Work out the finished part from the listing and answer in its coordinate system (mm). Face numbers are marked on the shaded views. A direction names the side the tool comes from. Give positions to 0.01 mm unless a question says otherwise; leave off trailing zeros. Order: outer loops, then holes, each group sorted by start corner. A loop starts at its lowest first (then second) coordinate and runs counter-clockwise, first axis right, second up. Notation, with made-up numbers: (79, 22) - (107, 22) arc R21 cw to (107, 53) - close; hole circle Ø7 at (60, -16). An arc over 180 degrees is marked (long way). Put each result on its own line as item: value.
```python
from build123d import *

# Parameters (mm, degrees)
F1_DEPTH = 25.4


with BuildPart() as f1:
    # F0 (on Right) → F1 (new body)
    with BuildSketch(Plane.YZ):
        with BuildLine():
            Line((-2.9690999484, -55.5171445012), (-30.2323300445, -55.5171445012))
            ThreePointArc((-30.2323300445, -55.5171445012), (-16.6007149965, -69.1487595492), (-2.9690999484, -55.5171445012))
        make_face()
        with BuildLine():
            ThreePointArc((1.0150714909, -55.5171445012), (14.1514278948, -68.6535009052), (27.2877842988, -55.5171445012))
            Line((27.2877842988, -55.5171445012), (1.0150714909, -55.5171445012))
        make_face()
        with BuildLine():
            ThreePointArc((-2.9690999484, -55.5171445012), (-16.6007149965, -41.8855294532), (-30.2323300445, -55.5171445012))
            Line((-30.2323300445, -55.5171445012), (-2.9690999484, -55.5171445012))
        make_face()
        with BuildLine():
            Line((1.0150714909, -55.5171445012), (27.2877842988, -55.5171445012))
            ThreePointArc((27.2877842988, -55.5171445012), (14.1514278948, -42.3807880973), (1.0150714909, -55.5171445012))
        make_face()
        with BuildLine():
            Line((-31.8407155573, -35.3785715997), (-31.8407155573, -55.5171445012))
            Line((-31.8407155573, -55.5171445012), (-30.2323300445, -55.5171445012))
            ThreePointArc((-30.2323300445, -55.5171445012), (-16.6007149965, -41.8855294532), (-2.9690999484, -55.5171445012))
            Line((-2.9690999484, -55.5171445012), (1.0150714909, -55.5171445012))
            ThreePointArc((1.0150714909, -55.5171445012), (14.1514278948, -42.3807880973), (27.2877842988, -55.5171445012))
            Line((27.2877842988, -55.5171445012), (44.3592844427, -55.5171445012))
            Line((44.3592844427, -55.5171445012), (44.3592844427, -35.3785715997))
            Line((44.3592844427, -35.3785715997), (-31.8407155573, -35.3785715997))
        make_face()
    extrude(amount=F1_DEPTH)


solid = f1.part
```
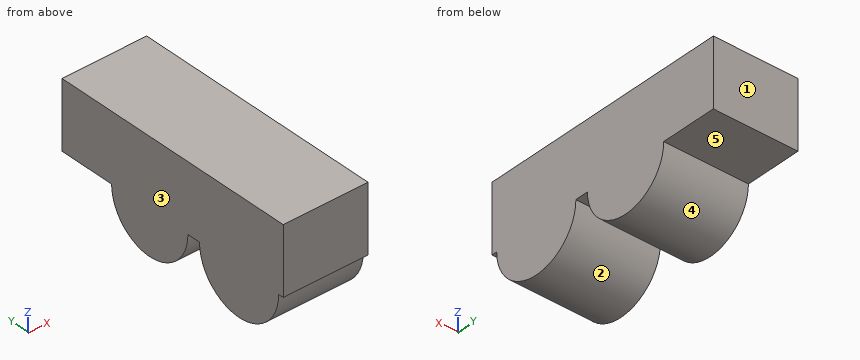
(1) Section D-D, the plane z = -59.5 is taken. Write down the section's boundary in (x, y), then the cut area to 3 significant figures.
Geometry check:
outline: (0, -29.64) - (25.4, -29.64) - (25.4, -3.56) - (0, -3.56) - close; (0, 1.63) - (25.4, 1.63) - (25.4, 26.67) - (0, 26.67) - close
area: 1,300 mm²
(2) Section C-C, the plane y = 38 is taken. Write down the section's boundary in (x, z), then the cut area to 3 significant figures.
Geometry check:
outline: (0, -55.52) - (25.4, -55.52) - (25.4, -35.38) - (0, -35.38) - close
area: 512 mm²
(3) A tool of negligible diameter and unlimited length cuts with its end or side. For the marked faces 4 and 5, from which of +Z, -Z, +X, -X, +Y, -Y can it reach the whole face along a straight path? Write none if from no direction.
Geometry check:
face 4: -Z, +X, -X
face 5: -Z, +X, -X, +Y
(4) Given pin 1 (5 mm diameter, centred on x = 9, y = 39, fed in from -Z); pin 2 (4.5 mm diameter, centred on x = 7.5, y = 0, fed in from -Z); pin 3 (8 mm diameter, centred on x = 10, z = -64, fed in from -Y), each flat-ended and moving along its own axis, determine where each tip first touches the part or whether it passes through.
Geometry check:
pin 1: stops at z = -55.52
pin 2: stops at z = -61.08
pin 3: stops at y = -29.47
(5) Section B-B, the plane z = -65 is taken. Write down the section's boundary in (x, y), then the cut area to 3 significant figures.
Geometry check:
outline: (0, -26.39) - (25.4, -26.39) - (25.4, -6.81) - (0, -6.81) - close; (0, 5.06) - (25.4, 5.06) - (25.4, 23.24) - (0, 23.24) - close
area: 959 mm²
(6) Determine the mould class of the marked faces 1, 2 and 3 for opening direction Y: pulls with the +Y half, pulls with the -Y half, needs draft (parallel to the pull), parting line crosses it, or undercut.
Geometry check:
face 1: pulls with the +Y half
face 2: undercut
face 3: needs draft
(7) Straight lines are drawn through the part: line 1 (Z direction, x = 1.25, y = 28); line 2 (Y direction, x = 12.25, z = -58.5); line 3 (Y direction, x = 11, z = -65). For each, find the intervals that lie inside material, in ascending order.
Geometry check:
line 1: z = -55.52 to -35.38
line 2: y = -29.9 to -3.3, 1.36 to 26.94
line 3: y = -26.39 to -6.81, 5.06 to 23.24
